For this review, take the finished solid that the model builds, in its own axes (mm). A direction names the side the tool comes from. Coordinates: 2 decimals unless noted, no trailing zeros. Write each loop counter-clockwise with the first axis right and the second up, starting at its lowest first coordinate (ties: lowest second). Pieces come first, ordered by that corner, then holes. Notation, with made-up numbers: (-38, 87) -> (19, 87) arc R10 ccw to (19, 100) -> close; hole circle Ø9 at (-17, 16). An arc over 180 degrees is marked (long way). One line per item, written item: value. Start each with the question number.
1) Add section D-D (y = 2.5). State the section outline as (x, z) points.
2) For probe 1 along Y at (x, z) = (0, -2.25); probe 2 along Z at (x, y) = (1.5, -10.75); probe 3 along Z at (x, y) = (-2.25, 1.5), list the stretches that pass through material, from the lowest coordinate up. Write a range as from..to.
3) Mouldability with a two-part tool opening along Y and no side actions: class faces 4 (the flat face through (0, -1, 0)), 5 (the flat face through (0, -9.8, 0)), 6 (the flat face through (0, 0, 8.5)) as released by +Y, released by -Y, zero draft, split by the parting line, or undercut.
4) For pin 1 Ø3.5 at (x, y) = (0, 5) entering from +Z; pin 2 Ø1.8 at (x, z) = (-0.5, 0) entering from -Y; pin 3 Ø0.5 at (y, z) = (3.5, 3.5) entering from -X, all flat-tipped, find the tip position at first contact; note any pin that passes through.
5) Add section A-A (z = -2). State the section outline as (x, y) points, and give its area (3 significant figures).
6) Add section C-C (x = 0). State the section outline as (y, z) points.
7) Add section B-B (z = 1). State the section outline as (x, y) points, and give its area (3 significant figures).
8) Machinability: for faces 1 (the flat face through (1.8, -7, 0)), 2 (the flat face through (-1.3, 4, 3)), 3 (the flat face through (0, 6, 5)), which of the approach directions +Z, -Z, +X, -X, +Y, -Y give a long, thin tool a straight path to every point of the face, cutting with its end or side? Answer none if there is none.
from build123d import *

# Parameters (mm, degrees)
SZKIC1_W                    = 7.6
SZKIC1_H                    = 5.6
DODANIE_WYCI_GNI_CIE1_DEPTH = 5
SZKIC2_R                    = 2.3
SZKIC2_W                    = 2.6
SZKIC2_H                    = 1.8
DODANIE_WYCI_GNI_CIE2_DEPTH = 5
SZKIC3_W                    = 3.6
SZKIC3_H                    = 7
DODANIE_WYCI_GNI_CIE3_DEPTH = 5
SZKIC4_R                    = 2.3
DODANIE_WYCI_GNI_CIE4_DEPTH = 8
SFAZOWANIE1_SIZE            = 3
SZKIC5_W                    = 3.5
SZKIC5_H                    = 5.6
DODANIE_WYCI_GNI_CIE5_DEPTH = 7.6
DODANIE_WYCI_GNI_CIE6_DEPTH = 3.6
SFAZOWANIE3_SIZE            = 1


with BuildPart() as part:
    # Szkic1 → Dodanie-wyciągnięcie1 (new body)
    with BuildSketch(Plane.XY):
        Rectangle(SZKIC1_W, SZKIC1_H)
    extrude(amount=DODANIE_WYCI_GNI_CIE1_DEPTH)

    # Szkic2 → Dodanie-wyciągnięcie2 (add)
    with BuildSketch(Plane.XY.offset(5)):
        with Locations((0, 6.497366596)):
            Circle(SZKIC2_R)
        with Locations((0, 3.7)):
            Rectangle(SZKIC2_W, SZKIC2_H)
    extrude(amount=-DODANIE_WYCI_GNI_CIE2_DEPTH)

    # Szkic3 → Dodanie-wyciągnięcie3 (add)
    with BuildSketch(Plane.XY.offset(5)):
        with Locations((0, -6.3)):
            Rectangle(SZKIC3_W, SZKIC3_H)
    extrude(amount=-DODANIE_WYCI_GNI_CIE3_DEPTH)

    # Szkic4 → Dodanie-wyciągnięcie4 (add)
    with BuildSketch(Plane(origin=(0, 0, 0), x_dir=(-1, 0, 0), z_dir=(0, 0, -1))):
        with Locations(Location((0, 6.497366596, 0), (0, 0, 235.58261129))):
            Circle(SZKIC4_R)
    extrude(amount=DODANIE_WYCI_GNI_CIE4_DEPTH)

    # Sfazowanie1
    sfazowanie1_edges = [part.edges().sort_by_distance(p)[0] for p in [
        (0, -9.8, 5),
    ]]
    chamfer(sfazowanie1_edges, length=SFAZOWANIE1_SIZE)

    # Szkic5 → Dodanie-wyciągnięcie5 (add)
    with BuildSketch(Plane(origin=(3.8, 0, 0), x_dir=(0, 0, -1), z_dir=(1, 0, 0))):
        with Locations((-6.75, 0)):
            Rectangle(SZKIC5_W, SZKIC5_H)
    extrude(amount=-DODANIE_WYCI_GNI_CIE5_DEPTH)

    # Szkic6 → Dodanie-wyciągnięcie6 (add)
    with BuildSketch(Plane.ZY.offset(1.8)):
        Polygon((0, -9.8), (-3, -9.8), (-3, -12.3), (-5.5, -12.3), (-5.5, -6.8), (0, -6.8), align=None)
    extrude(amount=-DODANIE_WYCI_GNI_CIE6_DEPTH)

    # Sfazowanie3
    sfazowanie3_edges = [part.edges().sort_by_distance(p)[0] for p in [
        (0, -2.8, 8.5),
        (0, 2.8, 8.5),
    ]]
    chamfer(sfazowanie3_edges, length=SFAZOWANIE3_SIZE)


solid = part.part
Numbers:
1. outline: (-3.8, 0) -> (3.8, 0) -> (3.8, 7.8) -> (-3.8, 7.8) -> close
2. probe 1: -9.8..-6.8, 4.2..8.8
2. probe 2: -5.5..-3
2. probe 3: 0..8.5
3. face 4: undercut
3. face 5: released by -Y
3. face 6: zero draft
4. pin 1: z = 5
4. pin 2: y = -9.8
4. pin 3: x = -1.3
5. outline: circle Ø4.6 at (0, 6.5); (-1.8, -9.8) -> (1.8, -9.8) -> (1.8, -6.8) -> (-1.8, -6.8) -> close
5. area: 27.4 mm²
6. outline: (-12.3, -5.5) -> (-6.8, -5.5) -> (-6.8, 0) -> (4.2, 0) -> (4.2, -8) -> (8.8, -8) -> (8.8, 5) -> (2.8, 5) -> (2.8, 7.5) -> (1.8, 8.5) -> (-1.8, 8.5) -> (-2.8, 7.5) -> (-2.8, 5) -> (-6.8, 5) -> (-9.8, 2) -> (-9.8, -3) -> (-12.3, -3) -> close
7. outline: (-3.8, -2.8) -> (-1.8, -2.8) -> (-1.8, -9.8) -> (1.8, -9.8) -> (1.8, -2.8) -> (3.8, -2.8) -> (3.8, 2.8) -> (1.3, 2.8) -> (1.3, 4.6) arc R2.3 ccw (long way) to (-1.3, 4.6) -> (-1.3, 2.8) -> (-3.8, 2.8) -> close
7. area: 88.3 mm²
8. face 1: +Z, -Z, +X, -Y
8. face 2: +Z, -Z, -X
8. face 3: +Z, +X, -X, +Y
